from build123d import *

# Parameters (mm, degrees)
SKETCH_1_R      = 1.7
EXTRUDE_1_DEPTH = 3


with BuildPart() as part:
    # 草图1 → 凸台-拉伸1 (new body)
    with BuildSketch(Plane(origin=(0, 0, 0), x_dir=(-1, 0, 0), z_dir=(0, 0, -1))):
        with BuildLine():
            Line((-15.441425808, 22.51249362), (-10.842226699, 17.91329451))
            ThreePointArc((-10.842226699, 17.91329451), (-10.278098339, 17.630675486), (-9.657048223, 17.742080476))
            ThreePointArc((-9.657048223, 17.742080476), (20.2, 0), (-9.657048223, -17.742080476))
            ThreePointArc((-9.657048223, -17.742080476), (-10.278098339, -17.630675486), (-10.842226699, -17.91329451))
            Line((-10.842226699, -17.91329451), (-15.441425808, -22.51249362))
            ThreePointArc((-15.441425808, -22.51249362), (-15.728277814, -23.329354358), (-15.270112446, -24.063949507))
            ThreePointArc((-15.270112446, -24.063949507), (28.5, 0), (-15.270112446, 24.063949507))
            ThreePointArc((-15.270112446, 24.063949507), (-15.728277814, 23.329354358), (-15.441425808, 22.51249362))
        make_face()
        with Locations(Location((0, 25, 0), (0, 0, 180))):
            Circle(SKETCH_1_R, mode=Mode.SUBTRACT)
        with Locations(Location((0, -25, 0), (0, 0, 180))):
            Circle(SKETCH_1_R, mode=Mode.SUBTRACT)
        with Locations(Location((21.650635095, 12.5, 0), (0, 0, 180))):
            Circle(SKETCH_1_R, mode=Mode.SUBTRACT)
        with Locations(Location((21.650635095, -12.5, 0), (0, 0, 180))):
            Circle(SKETCH_1_R, mode=Mode.SUBTRACT)
    extrude(amount=-EXTRUDE_1_DEPTH)


solid = part.part
Design review of the part built by this model. Coordinates are the model's own, in mm. A direction names the side the tool comes from. Round coordinates to 2 decimals unless told otherwise and drop trailing zeros. Loops run counter-clockwise (first coordinate to the right, second up) from the corner with the lowest first, then second, coordinate; pieces in that order, holes last. Notation, with made-up numbers: M 52,-9.5 L 87,-9.5 A22 cw 87,-2.5 Z; hole C 11.25,73.25 d6. An arc over 180 degrees is marked long. Answer as a JSON object with one key per item and string values.
Item 1: We need section A-A on x = 0. Give the boundary of the cut face in (y, z).
Answer sheet:
{"outline": "M -28.5,0 L -26.7,0 L -26.7,3 L -28.5,3 Z; M -23.3,0 L -20.2,0 L -20.2,3 L -23.3,3 Z; M 20.2,0 L 23.3,0 L 23.3,3 L 20.2,3 Z; M 26.7,0 L 28.5,0 L 28.5,3 L 26.7,3 Z"}
Item 2: We need section C-C on x = -4.5. Give the boundary of the cut face in (y, z).
Answer sheet:
{"outline": "M -28.14,0 L -19.69,0 L -19.69,3 L -28.14,3 Z; M 19.69,0 L 28.14,0 L 28.14,3 L 19.69,3 Z"}
Item 3: Machinability: for faces 5 (the flat face through (-21, 0, 0)), 6 (the flat face through (13.11, -20.18, 1.48)), 7 (the cylindrical face through (10.27, -17.63, 1.48)), which of the approach directions +Z, -Z, +X, -X, +Y, -Y give a long, thin tool a straight path to every point of the face, cutting with its end or side? Answer none if there is none.
Answer sheet:
{"face 5": "-Z, +X, -X, +Y, -Y", "face 6": "+Z, -Z, +X", "face 7": "+Z, -Z"}
Item 4: The part is to be moulded in two halves that separate along Y. For faces 1 (the flat face through (-21, 0, 3)), 2 (the cylindrical face through (15.73, -23.32, 1.48)), 3 (the cylindrical face through (-28.487, -0.852, 1.479)), 4 (the flat face through (13.174, 20.245, 1.479)), say which applies: pulls with the +Y half, pulls with the -Y half, needs draft (parallel to the pull), parting line crosses it, or undercut.
Answer sheet:
{"face 1": "needs draft", "face 2": "undercut", "face 3": "parting line crosses it", "face 4": "undercut"}
Item 5: We need section D-D on z = 1.9. Give the boundary of the cut face in (x, y), and give its area (3 significant figures).
Answer sheet:
{"outline": "M 9.66,-17.74 A20.2 cw long 9.66,17.74 A1 ccw 10.84,17.91 L 15.44,22.51 A1 ccw 15.27,24.06 A28.5 ccw long 15.27,-24.06 A1 ccw 15.44,-22.51 L 10.84,-17.91 A1 ccw Z; hole C -21.65,-12.5 d3.4; hole C -21.65,12.5 d3.4; hole C 0,-25 d3.4; hole C 0,25 d3.4", "area": "832 mm^2"}
Item 6: Clearance check with a flat-ended pin moving along its axis: P1, Ø1.5, axis at y = 21, z = 1, coming from the +X side. State where the tip first meets the part, or that it passes through.
Answer sheet:
{"P1": "stops at x = 14.68"}
Item 7: Wall thickness on L1, parallel to Y at x = 0, z = 1.05; L2, parallel to Y at x = 10, z = 2.85; L3, parallel to Y at x = -23, z = 1.35: over which ranges is each line inside the solid? List them lowest first. Write a range as from..to.
Answer sheet:
{"L1": "y = -28.5..-26.7, -23.3..-20.2, 20.2..23.3, 26.7..28.5", "L2": "y = -26.69..-17.63, 17.63..26.69", "L3": "y = -16.83..-13.53, -11.47..11.47, 13.53..16.83"}
Item 8: We need section B-B on y = -12.5. Give the boundary of the cut face in (x, z), and give its area (3 significant figures).
Answer sheet:
{"outline": "M -25.61,0 L -23.35,0 L -23.35,3 L -25.61,3 Z; M -19.95,0 L -15.87,0 L -15.87,3 L -19.95,3 Z", "area": "19.0 mm^2"}
